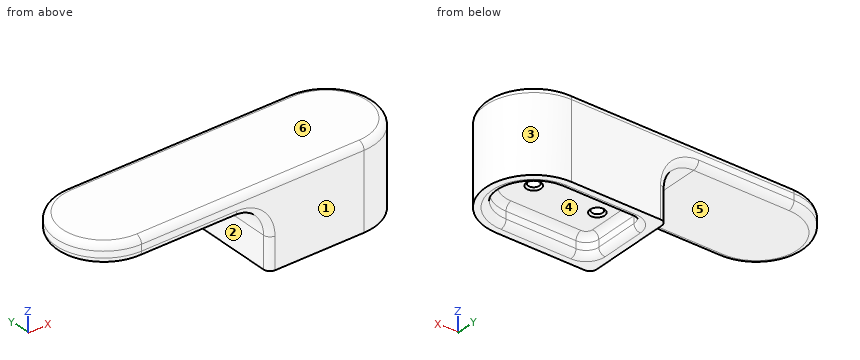
Autodesk Fusion 360 part; units mm, degrees
sketch "Sketch1" plane through (0, 0, 0) normal (0, 0, 1) x (1, 0, 0)
  line L0 (0, 0) -> (15, 0)
  line L1 (15, 0) -> (15, 15)
  line L2 (15, 15) -> (0, 15)
  line L3 (0, 15) -> (0, 0)
  circle A0 centre (15, 7.5) radius 7.5
  circle A1 centre (15, 7.5) radius 0.85
  circle A2 centre (5, 7.5) radius 0.85
  dimension "d1" = 15
  dimension "d2" = 15
  dimension "d3" = 1.7
  dimension "d4" = 10
  dimension "d5" = 7.5
  dimension "d6" = 1.7
extrude "Extrude1" add sketch "Sketch1" along normal blind 10 contours L0 L2 L3 A0 | L1 A0 A1 | L1 A0 A1
sketch "Sketch2" plane through (0, 0, 10) normal (0, 0, 1) x (-1, 0, 0)
  circle A0 centre (-5, -7.5) radius 0.85
  circle A1 centre (-15, -7.5) radius 0.85
  arc A2 (-15, 0) -> (-15, -15) centre (-15, -7.5) ccw
  line L0 (-15, -15) -> (0, -15)
  line L1 (0, -15) -> (0, 0)
  line L2 (0, 0) -> (-15, 0)
  line L3 (0, -15) -> (-15, -15)
  arc A3 (-15, 0) -> (-15, -15) centre (-15, -7.5) ccw
  line L4 (0, 0) -> (-15, 0)
  line L5 (0, -15) -> (0, 0)
  line L6 (0, 0) -> (20, 0)
  line L7 (20, 0) -> (20, -15)
  line L8 (20, -15) -> (0, -15)
  line L9 (0, -15) -> (0, 0)
  arc A4 (20, -15) -> (20, 0) centre (20, -7.5) ccw
  dimension "d9" = 20
  dimension "d10" = 15
extrude "Extrude2" add sketch "Sketch2" along normal blind 3 contours A0 | A1 | A2 L0 L1 L2 L3 A3 L4 L5 L9 | L1 L5 L6 L7 L8 L9 | L7 A4
fillet "Fillet1" radius 1 1 faces at (-1.6667, 5, 13)
fillet "Fillet2" radius 5 1 edges at (0, 7.5, 10)
fillet "Fillet3" radius 1 7 edges at (0, 15, 2.5) (-1.4645, 15, 8.5355) (-12.5, 15, 10) (-27.5, 7.5, 10) (-12.5, 0, 10) (-1.4645, 0, 8.5355) (0, 0, 2.5)
sketch "Sketch3" plane through (0, 0, 0) normal (0, 0, -1) x (1, 0, 0)
  arc A0 (1, 0) -> (0, -1) centre (1, -1) ccw
  line L0 (0, -1) -> (0, -14)
  arc A1 (0, -14) -> (1, -15) centre (1, -14) ccw
  line L1 (1, -15) -> (15, -15)
  arc A2 (15, -15) -> (15, 0) centre (15, -7.5) ccw
  line L2 (15, 0) -> (1, 0)
  line L3 (2, -2) -> (2, -13)
  line L4 (2, -13) -> (15, -13)
  arc A3 (15, -13) -> (15, -2) centre (15, -7.5) ccw
  line L5 (15, -2) -> (2, -2)
  circle A4 centre (5, -7.5) radius 0.85
  circle A5 centre (15, -7.5) radius 0.85
  dimension "d21" = -2
extrude "Extrude3" cut sketch "Sketch3" along normal blind 0 and the other way blind 3.15 contours L3 L4 A3 L5
fillet "Fillet4" radius 2 2 edges at (2, 13, 1.575) (2, 2, 1.575)
fillet "Fillet5" radius 1 6 edges at (2.5858, 12.4142, 3.15) (2, 7.5, 3.15) (2.5858, 2.5858, 3.15) (9.5, 2, 3.15) (20.5, 7.5, 3.15) (9.5, 13, 3.15)
fillet "Fillet6" radius 1 6 edges at (2.5858, 12.4142, 0) (2, 7.5, 0) (2.5858, 2.5858, 0) (9.5, 2, 0) (20.5, 7.5, 0) (9.5, 13, 0)
chamfer "Chamfer2" distance 0.3 angle 45 2 edges at (14.2075, 7.8074, 3.15) (4.2075, 7.8074, 3.15)
Source: CAD feature listing. Evaluate the final solid. Frame: model axes, mm. Face numbers are marked on the shaded views. A direction names the side the tool comes from. Coordinates: 2 decimals unless noted, no trailing zeros. Order: outer loops, then holes, each group sorted by start corner. A loop starts at its lowest first (then second) coordinate and runs counter-clockwise, first axis right, second up. Notation, with made-up numbers: (-40, 44.5) - (-5, 44.5) arc R24 cw to (-5, 63.5) - close; hole circle Ø8 at (-2.5, -4). An arc over 180 degrees is marked (long way). One line per item, written item: value.
1) Contact query for flat-ended pins moving along their axis: pin 1 (2 mm diameter, centred on x = 14, y = 12.5, fed in from -Z); pin 2 (4 mm diameter, centred on y = 6.5, z = 11, fed in from -X); pin 3 (1.3 mm diameter, centred on y = 6.5, z = 1.5, fed in from +X); pin 4 (1 mm diameter, centred on x = 15, y = 7.5, fed in from -Z). Output: stop coordinate, or through.
Computed values:
pin 1: stops at z = 0.13
pin 2: stops at x = -27.5
pin 3: stops at x = 22.49
pin 4: stops at z = 10
2) Cut plane A-A on x = 11. Output: boundary loops of the cut face in (y, z), plus the area to 3 significant figures.
Computed values:
outline: (0, 0) - (1, 0) arc R1 ccw to (2, 1) - (2, 2.15) arc R1 cw to (3, 3.15) - (12, 3.15) arc R1 cw to (13, 2.15) - (13, 1) arc R1 ccw to (14, 0) - (15, 0) - (15, 12) arc R1 ccw to (14, 13) - (1, 13) arc R1 ccw to (0, 12) - close
area: 160 mm^2
3) Cut plane D-D on x = 5. Output: boundary loops of the cut face in (y, z), plus the area to 3 significant figures.
Computed values:
outline: (0, 0) - (1, 0) arc R1 ccw to (2, 1) - (2, 2.15) arc R1 cw to (3, 3.15) - (6.35, 3.15) - (6.65, 3.45) - (6.65, 10) - (8.35, 10) - (8.35, 3.45) - (8.65, 3.15) - (12, 3.15) arc R1 cw to (13, 2.15) - (13, 1) arc R1 ccw to (14, 0) - (15, 0) - (15, 12) arc R1 ccw to (14, 13) - (1, 13) arc R1 ccw to (0, 12) - close
area: 148 mm^2
4) Cut plane C-C on x = -9.5. Output: boundary loops of the cut face in (y, z), plus the area to 3 significant figures.
Computed values:
outline: (0, 11) arc R1 ccw to (1, 10) - (14, 10) arc R1 ccw to (15, 11) - (15, 12) arc R1 ccw to (14, 13) - (1, 13) arc R1 ccw to (0, 12) - close
area: 44.1 mm^2
5) Mould query, pull axis X, two halves, no side actions, for the marked faces 1, 2, 3 and 4. Classes: released by +X, released by -X, zero draft, split by the parting line, or undercut.
Computed values:
face 1: zero draft
face 2: released by -X
face 3: released by +X
face 4: undercut
6) Reachability of the marked faces 5 and 6 from +Z, -Z, +X, -X, +Y, -Y: full face, straight path, thin tool, end or side. Return the list, or none.
Computed values:
face 5: -Z, -X, +Y, -Y
face 6: +Z, +X, -X, +Y, -Y
7) Cut plane B-B on z = 9.5. State how many separate pieces and enclosed holes the cut face has, plus the area to 3 significant figures.
Computed values:
separate pieces: 1
enclosed holes: 2
area: 350 mm^2
8) Ray query, line 1 (X direction, y = 7.5, z = 5); line 2 (Y direction, x = 15, z = 5.75); line 3 (X direction, y = 7.5, z = 6.25). Return the intervals inside material, ascending. Write a range as [from, to].
Computed values:
line 1: x = [0, 4.15], [5.85, 14.15], [15.85, 22.5]
line 2: y = [0, 6.65], [8.35, 15]
line 3: x = [-0.16, 4.15], [5.85, 14.15], [15.85, 22.5]
